from build123d import *

# Parameters (mm, degrees)
SKETCH1_R           = 1.7018
SKETCH1_R_2         = 3.2385
BOSS_EXTRUDE1_DEPTH = 3.175


with BuildPart() as part:
    # Sketch1 → Boss-Extrude1 (new body)
    with BuildSketch(Plane(origin=(0, 0, 0), x_dir=(1, 0, 0), z_dir=(0, 1, 0))):
        with BuildLine():
            Line((-26.385767095, 2.692431218), (-9.650546347, -0.397020276))
            ThreePointArc((-9.650546347, -0.397020276), (-8.345625907, -1.243134279), (-8.021200765, -2.76414532))
            Line((-8.021200765, -2.76414532), (-10.188427932, -14.503777784))
            Line((-10.188427932, -14.503777784), (-10.188427932, -25.895050365))
            ThreePointArc((-10.188427932, -25.895050365), (-9.718255056, -27.194942681), (-8.525317662, -27.893285678))
            Line((-8.525317662, -27.893285678), (3.434770775, -30.101210727))
            ThreePointArc((3.434770775, -30.101210727), (4.798418745, -29.874833209), (5.701723859, -28.828495578))
            Line((5.701723859, -28.828495578), (9.768947258, -18.188063969))
            Line((9.768947258, -18.188063969), (11.936174425, -6.448431504))
            ThreePointArc((11.936174425, -6.448431504), (12.782288428, -5.143511064), (14.303299469, -4.819085921))
            Line((14.303299469, -4.819085921), (14.67796859, -4.888252746))
            ThreePointArc((14.67796859, -4.888252746), (19.245190129, -7.849651756), (20.380678129, -13.173190399))
            Line((20.380678129, -13.173190399), (16.362085627, -34.941466341))
            ThreePointArc((16.362085627, -34.941466341), (13.400686617, -39.50868788), (8.077147974, -40.64417588))
            Line((8.077147974, -40.64417588), (-32.986587711, -33.063491917))
            ThreePointArc((-32.986587711, -33.063491917), (-37.064464086, -30.419385658), (-38.078292657, -25.666226155))
            Line((-38.078292657, -25.666226155), (-33.783032856, -2.399273728))
            ThreePointArc((-33.783032856, -2.399273728), (-31.138926597, 1.678602647), (-26.385767095, 2.692431218))
        make_face()
        with Locations((12.145909657, -21.752201671)):
            Circle(SKETCH1_R, mode=Mode.SUBTRACT)
        with Locations((-13.681281765, -16.984301904)):
            Circle(SKETCH1_R, mode=Mode.SUBTRACT)
        with Locations((-27.68794209, -15.55442008)):
            Circle(SKETCH1_R_2, mode=Mode.SUBTRACT)
    extrude(amount=BOSS_EXTRUDE1_DEPTH)


solid = part.part
Could you check a few things on this model? Use its own coordinates, in mm. A direction names the side the tool comes from. Coordinates: 2 decimals unless noted, no trailing zeros. Write each loop counter-clockwise with the first axis right and the second up, starting at its lowest first coordinate (ties: lowest second). Pieces come first, ordered by that corner, then holes. Notation, with made-up numbers: (52.5, 0) - (106.5, 0) arc R15 ccw to (106.5, 29) - close; hole circle Ø7 at (-23, 63). An arc over 180 degrees is marked (long way). Put each result on its own line as item: value. Start each with the question number.
Q1. I want a section at B-B on y = 2.3. Write out the boundary of the cut face in (x, z), plus the area to 3 significant figures.
Q2. I want a section at D-D on z = 38. Write out the boundary of the cut face in (x, y) (3 decimals).
Q3. Please list where these lines run through material, in increasing order: L1, parallel to X at y = 2.25, z = 18; L2, parallel to Z at x = -12.5, y = 2.35; L3, parallel to X at y = 0.8, z = 9.
Q4. I'm going to push flat-ended pins straight in: P1, Ø5, axis at x = -5.5, z = 20.5, coming from the -Y side; P2, Ø1.6, axis at y = 1, z = 19, coming from the +X side. Where does each tip first touch, or does it pass through?
Q5. Thinking about a two-plate mould opening in X: for faces 4 (the cylindrical face through (-9.73, 1.57, 27.18)), 5 (the cylindrical face through (-37.02, 1.57, 30.48)), 6 (the flat face through (-18.14, 1.57, -1.17)), which applies, pulls with the +X half, pulls with the -X half, needs draft (parallel to the pull), parting line crosses it, or undercut?
Q6. I want a section at A-A on x = -28.5. Write out the boundary of the cut face in (y, z) (3 decimals).
Q7. I want a section at C-C on x = -17. Write out the boundary of the cut face in (y, z) (3 decimals).
Q8. Which directions (+Z, -Z, +X, -X, +Y, -Y) give clear straight access to the entire face, cutting with the end or side of a thin tool? Please do faces 1 (the flat face through (-9.1, 1.6, 8.6)), 2 (the flat face through (-15, 3.175, 19)), 3 (the flat face through (10.837, 1.565, 12.4)).
Checks:
1. outline: (-38.08, 25.67) - (-33.78, 2.4) arc R6.35 ccw to (-26.39, -2.69) - (-9.65, 0.4) arc R2.03 ccw to (-8.02, 2.76) - (-10.19, 14.5) - (-10.19, 25.9) arc R2.03 cw to (-8.53, 27.89) - (3.43, 30.1) arc R2.03 cw to (5.7, 28.83) - (9.77, 18.19) - (11.94, 6.45) arc R2.03 ccw to (14.3, 4.82) - (14.68, 4.89) arc R7.11 ccw to (20.38, 13.17) - (16.36, 34.94) arc R7.11 ccw to (8.08, 40.64) - (-32.99, 33.06) arc R6.35 ccw to start; hole circle Ø6.48 at (-27.69, 15.55); hole circle Ø3.4 at (-13.68, 16.98); hole circle Ø3.4 at (12.15, 21.75)
1. area: 1,400 mm²
2. outline: (-6.246, 0) - (14.995, 0) - (14.995, 3.175) - (-6.246, 3.175) - close
3. L1: -36.66 to -29.81, -25.56 to -15.05, -12.32 to -10.19, 9.8 to 19.49
3. L2: -0.13 to 15.76, 18.21 to 36.85
3. L3: -35 to -9.17, 11.47 to 19.89
4. P1: through
4. P2: x = 19.45
5. face 4: undercut
5. face 5: pulls with the -X half
5. face 6: pulls with the +X half
6. outline: (0, -2.725) - (3.175, -2.725) - (3.175, 12.419) - (0, 12.419) - close; (0, 18.689) - (3.175, 18.689) - (3.175, 33.892) - (0, 33.892) - close
7. outline: (0, -0.96) - (3.175, -0.96) - (3.175, 36.015) - (0, 36.015) - close
8. face 1: +Y, -Y
8. face 2: +Z, -Z, +X, -X, +Y
8. face 3: -Z, +Y, -Y
